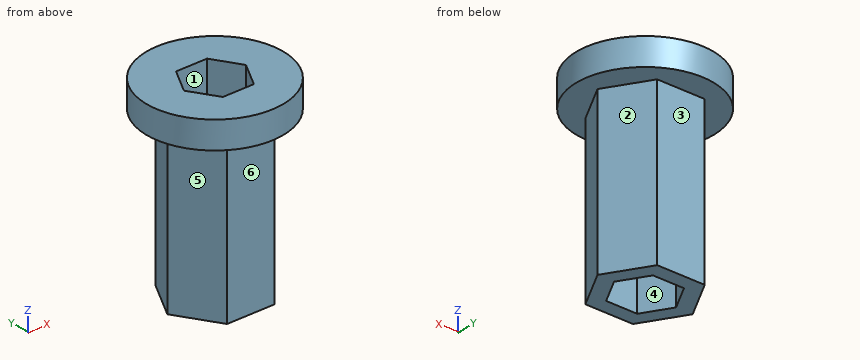
```python
from build123d import *

# Parameters (mm, degrees)
PAD_DEPTH     = 14
SKETCH001_R   = 5
SKETCH001_R_2 = 2.678441
PAD001_DEPTH  = 2


with BuildPart() as part:
    # Sketch → Pad (new body)
    with BuildSketch(Plane.XY):
        Polygon((3.585345, 0), (1.792673, 3.105), (-1.792673, 3.105), (-3.585345, 0), (-1.792673, -3.105), (1.792673, -3.105), align=None)
        Polygon((-2.338269, 0), (-1.169134, -2.025), (1.169134, -2.025), (2.338269, 0), (1.169134, 2.025), (-1.169134, 2.025), align=None, mode=Mode.SUBTRACT)
    extrude(amount=PAD_DEPTH)

    # Sketch001 (on Face14 of Pad) → Pad001 (join)
    with BuildSketch(Plane.XY.offset(14)):
        Circle(SKETCH001_R)
        Circle(SKETCH001_R_2, mode=Mode.SUBTRACT)
    extrude(amount=-PAD001_DEPTH)


solid = part.part
```
Geometry check sheet. Reference: the model listing, model coordinates, mm. Face numbers are marked on the shaded views. A direction names the side the tool comes from. Coordinates: 2 decimals unless noted, no trailing zeros. Write each loop counter-clockwise with the first axis right and the second up, starting at its lowest first coordinate (ties: lowest second). Pieces come first, ordered by that corner, then holes. Notation, with made-up numbers: M 23,50.5 L 43,50.5 A15 ccw 43,77.5 Z; hole C -17.5,36 d6. An arc over 180 degrees is marked long. One line per item, written item: value. Start each with the question number.
(1) Depth check by flat-ended pin: pin 1 (2.5 mm diameter, centred on x = -0.5, z = 9.5, fed in from +Y) (3 decimals); pin 2 (3 mm diameter, centred on y = -3, z = 4.5, fed in from +X); pin 3 (1.2 mm diameter, centred on x = 0.5, z = 8.5, fed in from -Y) (3 decimals). Enter the tip coordinate at first touch or a pass-through.
(2) Sectioned sample at B-B, the plane y = -0.25. Enter the section's corners in (x, z), and give its area (3 significant figures).
(3) Tool access check on the marked faces 4, 5 and 6. Record the directions out of +Z, -Z, +X, -X, +Y, -Y that give a thin tool (end or side, any length) a straight path to the whole face; none if there is none.
(4) Sectioned sample at C-C, the plane z = 7.75. Enter the section's corners in (x, y) (3 decimals), and give its area (3 significant figures).
(5) Scan lines: line 1 along Y through (x, z) = (0.5, 8.75) (3 decimals); line 2 along Z through (x, y) = (1.75, 4.25); line 3 along X through (y, z) = (0.5, 6). Record each from-to range of solid material in increasing order. Write a range as [from, to].
(6) Sectioned sample at A-A, the plane x = 0. Enter the section's corners in (y, z) (3 decimals), and give its area (3 significant figures).
(7) Release check for a two-part mould opening along X. For the marked faces 1, 2 and 3 record: released by +X, released by -X, zero draft, split by the parting line, or undercut.
(8) Sectioned sample at D-D, the plane y = -2.75. Enter the section's corners in (x, z), and give its area (3 significant figures).
Filled sheet:
1. pin 1: y = 3.105
1. pin 2: x = 2.72
1. pin 3: y = -3.105
2. outline: M -4.99,12 L -3.44,12 L -3.44,0 L -2.19,0 L -2.19,14 L -4.99,14 Z; M 2.19,0 L 3.44,0 L 3.44,12 L 4.99,12 L 4.99,14 L 2.19,14 Z
2. area: 41.1 mm²
3. face 4: +Z, -Z
3. face 5: -Z, -X, -Y
3. face 6: -Z, +X, -X, -Y
4. outline: M -3.585,0 L -1.793,-3.105 L 1.793,-3.105 L 3.585,0 L 1.793,3.105 L -1.793,3.105 Z; hole M -2.338,0 L -1.169,-2.025 L 1.169,-2.025 L 2.338,0 L 1.169,2.025 L -1.169,2.025 Z
4. area: 19.2 mm²
5. line 1: [-3.105, -2.025], [2.025, 3.105]
5. line 2: [12, 14]
5. line 3: [-3.3, -2.05], [2.05, 3.3]
6. outline: M -5,12 L -3.105,12 L -3.105,0 L -2.025,0 L -2.025,14 L -5,14 Z; M 2.025,0 L 3.105,0 L 3.105,12 L 5,12 L 5,14 L 2.025,14 Z
6. area: 37.8 mm²
7. face 1: undercut
7. face 2: released by +X
7. face 3: zero draft
8. outline: M -4.18,12 L -2,12 L -2,0 L 2,0 L 2,12 L 4.18,12 L 4.18,14 L -4.18,14 Z
8. area: 64.6 mm²
